```python
from build123d import *

# Parameters (mm, degrees)
F0_R      = 12.672559
F1_DEPTH  = 25.4
F2_R      = 5.08
F3_R      = 5.08
F4_R      = 3.609699
F5_DEPTH  = 50.8
F5_FACE_R = 3.609699
F6_DEPTH  = 101.6


with BuildPart() as f1:
    # F0 (on Front) → F1 (new body)
    with BuildSketch(Plane.XZ):
        Circle(F0_R)
    extrude(amount=F1_DEPTH)

    # F2
    f2_edges = [f1.edges().sort_by_distance(p)[0] for p in [
        (-12.672559, -25.4, 0),
    ]]
    fillet(f2_edges, radius=F2_R)

    # F3
    f3_edges = [f1.edges().sort_by_distance(p)[0] for p in [
        (-12.672559, 0, 0),
    ]]
    fillet(f3_edges, radius=F3_R)

    # F4 (on Right) → F5 (cut)
    with BuildSketch(Plane.YZ):
        with Locations((-12.31988, 4.152768)):
            Circle(F4_R)
    extrude(amount=-F5_DEPTH, mode=Mode.SUBTRACT)

    # F5_face (on face) → F6 (cut)
    with BuildSketch(Plane(origin=(0, -12.31988, 4.152768), x_dir=(0, 1, 0), z_dir=(-1, 0, 0))):
        Circle(F5_FACE_R)
    extrude(amount=-F6_DEPTH, mode=Mode.SUBTRACT)


solid = f1.part
```
CAD build for the part. Positions are in the model's coordinates, mm. Round coordinates to 2 decimals unless told otherwise and drop trailing zeros. Order: outer loops, then holes, each group sorted by start corner. A loop starts at its lowest first (then second) coordinate and runs counter-clockwise, first axis right, second up.
Item 1: Pin check, flat tips, straight feed: pin 1 (2 mm diameter, centred on x = -7.5, z = -7, fed in from +Y); pin 2 (1 mm diameter, centred on x = 1.5, y = -12.5, fed in from -Z); pin 3 (8 mm diameter, centred on x = -7, y = -8.5, fed in from +Z). Stop position of each tip, or through.
Item 2: Probe line 1 along Z through (x, y) = (-1, -10); line 2 along Z through (x, y) = (9.75, -12); line 3 along Y through (x, z) = (-7.25, 2.25). List the from-to ranges inside material, lowest first.
Item 3: Saw through at B-B on x = 0. Write the cut outline in (y, z).
Item 4: Saw through at C-C on y = -7.75. Write the cut outline in (x, z), then the cut area to 3 significant figures.
Item 5: Saw through at D-D on y = -2.25. Write the cut outline in (x, z).
Item 6: Saw through at A-A on z = 0. Write the cut outline in (x, y).
Reported:
1. pin 1: stops at y = -0.28
1. pin 2: stops at z = -12.63
1. pin 3: stops at z = 12.31
2. line 1: z = -12.63 to 1.39, 6.92 to 12.63
2. line 2: z = -8.1 to 0.56, 7.75 to 8.1
2. line 3: y = -25.4 to -15.39, -9.25 to 0
3. outline: (-25.4, -7.59) arc R5.08 ccw to (-20.32, -12.67) - (-5.08, -12.67) arc R5.08 ccw to (0, -7.59) - (0, 7.59) arc R5.08 ccw to (-5.08, 12.67) - (-20.32, 12.67) arc R5.08 ccw to (-25.4, 7.59) - close; hole circle Ø7.22 at (-12.32, 4.15)
4. outline: circle Ø25.35 at (0, 0)
4. area: 505 mm2
5. outline: circle Ø23.62 at (0, 0)
6. outline: (-12.67, -20.32) arc R5.08 ccw to (-7.59, -25.4) - (7.59, -25.4) arc R5.08 ccw to (12.67, -20.32) - (12.67, -5.08) arc R5.08 ccw to (7.59, 0) - (-7.59, 0) arc R5.08 ccw to (-12.67, -5.08) - close
